from build123d import *

# Parameters (mm, degrees)
F1_DEPTH  = 45
F2_W      = 13.4
F2_H      = 19.6
F3_DEPTH  = 3
F5_DEPTH  = 1
F7_W      = 125.609561801
F7_H      = 4.575594794
F8_DEPTH  = 1.5
F9_W      = 1.9871633053
F9_H      = 26.1965505779
F10_DEPTH = 16
F6_R      = 2
F11_DEPTH = 9.4


with BuildPart() as f1:
    # F0 (on Top) → F1 (new body)
    with BuildSketch(Plane.XY):
        Polygon((-64, 0), (-62.5, 0), (-62.5, 67), (62.5, 67), (62.5, 0), (64, 0), (64, 68.5), (-64, 68.5), align=None)
    extrude(amount=F1_DEPTH)

    # F2 (on face) → F3 (cut, symmetric)
    with BuildSketch(Plane(origin=(-64, 0, 0), x_dir=(0, -1, 0), z_dir=(-1, 0, 0))):
        with Locations((-56.0214279117, 29.8)):
            Rectangle(F2_W, F2_H)
    extrude(amount=F3_DEPTH, both=True, mode=Mode.SUBTRACT)

    # F4 (on face) → F5 (join)
    with BuildSketch(Plane.XY.offset(45)):
        Polygon((-42.12194103, 67), (-62.5, 67), (-62.5, 46.62194103), align=None)
        Polygon((62.5, 67), (42.12194103, 67), (62.5, 46.62194103), align=None)
    extrude(amount=-F5_DEPTH)

    # F7 (on face) → F8 (join)
    with BuildSketch(Plane.XY.offset(45)):
        with Locations((0.1741200686, 2.287797397)):
            Rectangle(F7_W, F7_H)
    extrude(amount=-F8_DEPTH)

    # F9 (on face) → F10 (join)
    with BuildSketch(Plane.XZ.offset(-67)):
        with Locations((59.5064183474, 13.0982752889)):
            Rectangle(F9_W, F9_H)
    extrude(amount=F10_DEPTH)

    # F6 (on face) → F11 (cut, symmetric)
    with BuildSketch(Plane.YZ.offset(64)):
        with Locations((58.5, 15)):
            Circle(F6_R)
    extrude(amount=F11_DEPTH, both=True, mode=Mode.SUBTRACT)


solid = f1.part
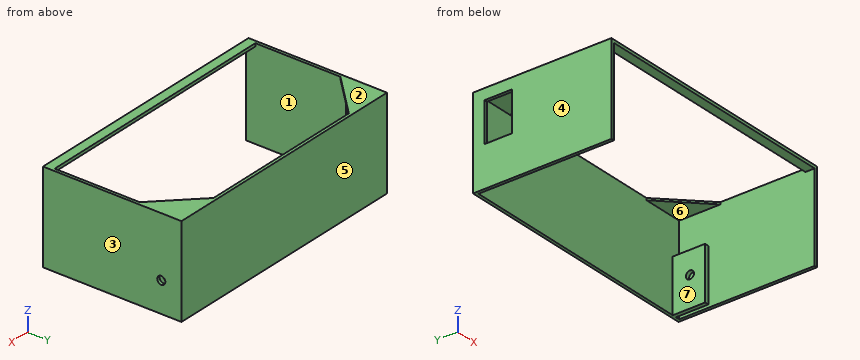
Part model, mm, in its own coordinate system. Face numbers are marked on the shaded views. A direction names the side the tool comes from. Give positions to 0.01 mm unless a question says otherwise; leave off trailing zeros. Loops run counter-clockwise (first coordinate to the right, second up) from the corner with the lowest first, then second, coordinate; pieces in that order, holes last. Notation, with made-up numbers: M 65,11.5 L 93,11.5 A31 ccw 93,35.5 Z; hole C 75.25,28.25 d9. An arc over 180 degrees is marked long. Put each result on its own line as item: value. Start each with the question number.
1) Probe probe 1 along Z at (x, y) = (59.8, 58.5); probe 2 along X at (y, z) = (60.5, 18); probe 3 along X at (y, z) = (40, 37). List the from-to ranges inside material, lowest first.
2) Pull direction X, two halves, no side cores. Call the marked faces 1, 2, 3 and 4: +X half, -X half, draft (parallel to the pull), parting line (faces both ways), or undercut.
3) Saw through at C-C (z = 15). List the corners of the cut face in (x, y).
4) Saw through at B-B (y = 39). List the corners of the cut face in (x, z).
5) Flat gauge pins, fed straight in: pin 1 (3 mm diameter, centred on y = 53, z = 26.5, fed in from -X); pin 2 (1 mm diameter, centred on x = -36, z = 21.5, fed in from -Y); pin 3 (2.5 mm diameter, centred on x = -14.5, y = 2.5, fed in from -Z). Where does each tip first touch, or does it go through?
6) 3-axis set-ups, long thin cutter, end or side, ignore diameter. For the marked faces 5, 6 and 7: which of +Z, -Z, +X, -X, +Y, -Y reach the whole face in a straight line?
7) Saw through at A-A (x = -30). List the corners of the cut face in (y, z).
8) Saw through at D-D (y = 58.5). List the corners of the cut face in (x, z), then the cut area to 3 significant figures.
Numbers:
1. probe 1: 0 to 13, 17 to 26.2, 44 to 45
1. probe 2: -64 to -62.5, 58.51 to 60.5, 62.5 to 64
1. probe 3: -64 to -62.5, 62.5 to 64
2. face 1: undercut
2. face 2: draft
2. face 3: +X half
2. face 4: -X half
3. outline: M -64,0 L -62.5,0 L -62.5,67 L 58.51,67 L 58.51,60.5 L 60.5,60.5 L 60.5,67 L 62.5,67 L 62.5,60.5 L 64,60.5 L 64,68.5 L -64,68.5 Z; M 58.51,51 L 60.5,51 L 60.5,56.5 L 58.51,56.5 Z; M 62.5,0 L 64,0 L 64,56.5 L 62.5,56.5 Z
4. outline: M -64,0 L -62.5,0 L -62.5,45 L -64,45 Z; M 62.5,0 L 64,0 L 64,45 L 62.5,45 Z
5. pin 1: x = 58.51
5. pin 2: y = 67
5. pin 3: z = 43.5
6. face 5: +Z, -Z, +X, -X, +Y
6. face 6: none
6. face 7: -Z, -Y
7. outline: M 0,43.5 L 4.58,43.5 L 4.58,45 L 0,45 Z; M 67,0 L 68.5,0 L 68.5,45 L 67,45 Z
8. outline: M -64,0 L -62.5,0 L -62.5,20 L -64,20 Z; M -64,39.6 L -62.5,39.6 L -62.5,44 L -50.62,44 L -50.62,45 L -64,45 Z; M 50.62,44 L 62.5,44 L 62.5,17 L 64,17 L 64,45 L 50.62,45 Z; M 58.51,0 L 60.5,0 L 60.5,13 L 58.51,13 Z; M 58.51,17 L 60.5,17 L 60.5,26.2 L 58.51,26.2 Z; M 62.5,0 L 64,0 L 64,13 L 62.5,13 Z
8. area: 167 mm^2
